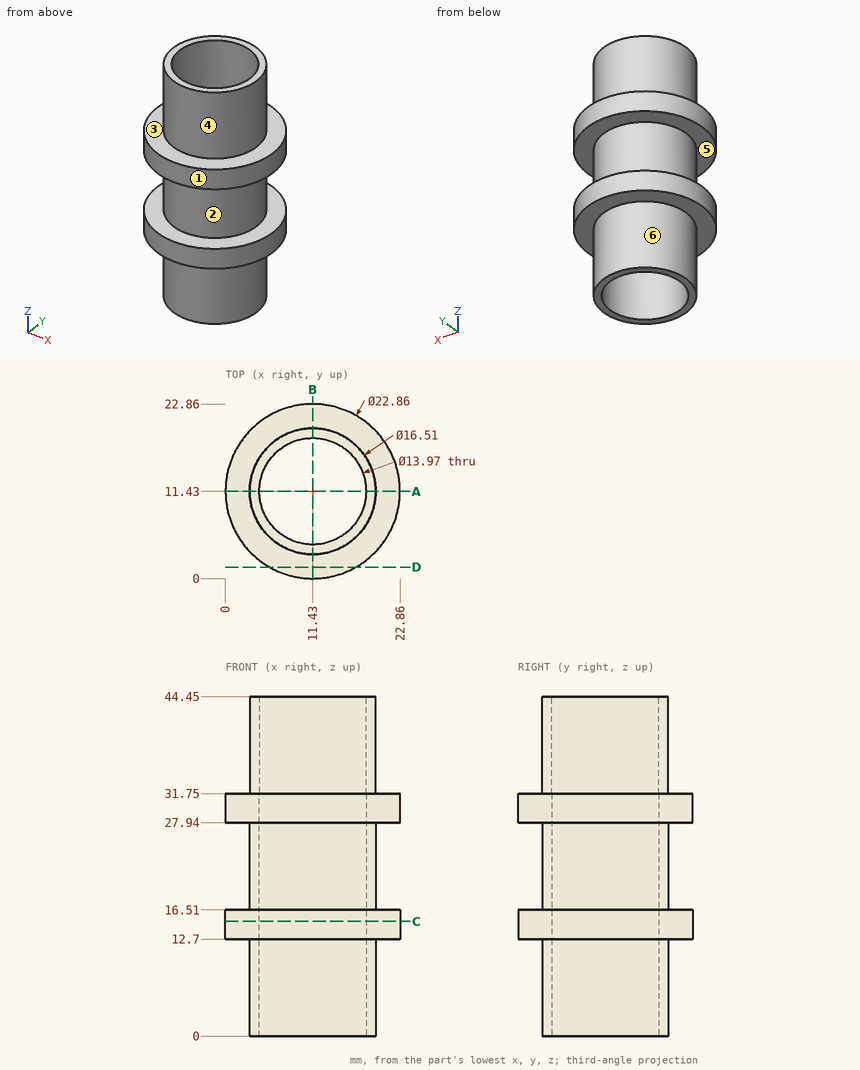
Part print with two shaded views. Sizes in mm from the minimum x, y, z corner. A direction names the side the tool comes from. Coordinates: 2 decimals unless noted, no trailing zeros. Loops run counter-clockwise (first coordinate to the right, second up) from the corner with the lowest first, then second, coordinate; pieces in that order, holes last. Notation, with made-up numbers: M 1.5,43.5 L 9.5,43.5 A13 cw 9.5,66.5 Z; hole C 33.5,-0.75 d3. An arc over 180 degrees is marked long. Use CSV: the item, a comma, the result in double quotes. Start each with the question number.
1. Two-plate mould, pull along Z, no slides. Class the marked faces 1, 2 and 3: pulls with the +Z half, pulls with the -Z half, needs draft (parallel to the pull), parting line crosses it, or undercut.
2. Probe probe 1 along Z at (x, y) = (10.75, 21); probe 2 along Y at (x, z) = (11.43, 8.75) (3 decimals); probe 3 along X at (y, z) = (11.75, 22.5). List the from-to ranges inside material, lowest first. Write a range as [from, to].
3. Band-saw the part on C-C, the plane z = 15. List the corners of the cut face in (x, y) (3 decimals).
4. Flat gauge pins, fed straight in: pin 1 (3 mm diameter, centred on x = 18, z = 25, fed in from -Y); pin 2 (1 mm diameter, centred on y = 19, z = 34, fed in from -X); pin 3 (1.5 mm diameter, centred on y = 13.5, z = 27, fed in from -X). Where does each tip first touch, or does it go through?
5. Tool access for the marked faces 4, 5 and 6: list every direction of +Z, -Z, +X, -X, +Y, -Y with a clear straight run to the whole face (end or side of a thin tool).
6. Band-saw the part on A-A, the plane y = 11.43. List the corners of the cut face in (x, z) (3 decimals), then the cut area to 3 significant figures.
7. Band-saw the part on D-D, the plane y = 1.5. List the corners of the cut face in (x, z), then the cut area to 3 significant figures.
Entries:
1,face 1,"needs draft"
1,face 2,"undercut"
1,face 3,"pulls with the +Z half"
2,probe 1,"z = [12.7, 16.51], [27.94, 31.75]"
2,probe 2,"y = [3.175, 4.445], [18.415, 19.685]"
2,probe 3,"x = [3.18, 4.45], [18.41, 19.68]"
3,outline,"C 11.43,11.43 d22.86; hole C 11.43,11.43 d13.97"
4,pin 1,"stops at y = 4.92"
4,pin 2,"stops at x = 7.17"
4,pin 3,"stops at x = 3.28"
5,face 4,"+Z"
5,face 5,"none"
5,face 6,"-Z"
6,outline,"M 0,12.7 L 3.175,12.7 L 3.175,0 L 4.445,0 L 4.445,44.45 L 3.175,44.45 L 3.175,31.75 L 0,31.75 L 0,27.94 L 3.175,27.94 L 3.175,16.51 L 0,16.51 Z; M 18.415,0 L 19.685,0 L 19.685,12.7 L 22.86,12.7 L 22.86,16.51 L 19.685,16.51 L 19.685,27.94 L 22.86,27.94 L 22.86,31.75 L 19.685,31.75 L 19.685,44.45 L 18.415,44.45 Z"
6,area,"161 mm2"
7,outline,"M 5.77,12.7 L 17.09,12.7 L 17.09,16.51 L 5.77,16.51 Z; M 5.77,27.94 L 17.09,27.94 L 17.09,31.75 L 5.77,31.75 Z"
7,area,"86.3 mm2"
